Autodesk Inventor part; units mm, degrees
ref_plane "YZ Plane" through (0, 0, 0) normal (1, 0, 0) x (0, 1, 0)
ref_plane "XZ Plane" through (0, 0, 0) normal (0, 1, 0) x (-1, 0, 0)
ref_plane "XY Plane" through (0, 0, 0) normal (0, 0, 1) x (1, 0, 0)
sketch "Sketch1" plane through (0, 0, 0) normal (0, 0, 1) x (1, 0, 0)
  line L0 (0, 40) -> (34.641, -20)
  line L1 (34.641, -20) -> (-34.641, -20)
  line L2 (-34.641, -20) -> (0, 40)
  circle A0 centre (0, 0) radius 1
  dimension "d0" = 2
  dimension "d1" = 20
extrude "Extrusion1" add sketch "Sketch1" along normal blind 5.66
sketch "Sketch2" plane through (0, 0, 5.66) normal (0, 0, 1) x (1, 0, 0)
  circle A0 centre (0, 0) radius 1
  line L0 (-34.641, -20) -> (34.641, -20)
  line L1 (0, -1) -> (0, 0)
  line L2 (-2.83, -11.66) -> (-2.83, -20)
  line L3 (2.83, -11.66) -> (2.83, -20)
  line L4 (2.83, -11.66) -> (-2.83, -11.66)
  point P0 (0, -20)
  dimension "d15" = 8.34
  dimension "d16" = 2.83
  dimension "d17" = 2.83
extrude "Extrusion2" cut sketch "Sketch2" against normal blind 8.625
pattern_circular "Circular Pattern1" count 3 over 360 about axis through (0, 0, 0) along (0, 0, 1) of "Extrusion2"
chamfer "Chamfer1" distance 10 angle 45 3 edges at (34.641, -20, 2.83) (-34.641, -20, 2.83) (0, 40, 2.83)
fillet "Fillet1" radius 2 6 edges at (-29.641, -11.3397, 2.83) (-24.641, -20, 2.83) (-5, 31.3397, 2.83) (5, 31.3397, 2.83) (29.641, -11.3397, 2.83) (24.641, -20, 2.83)
properties part number "Lower Platform"
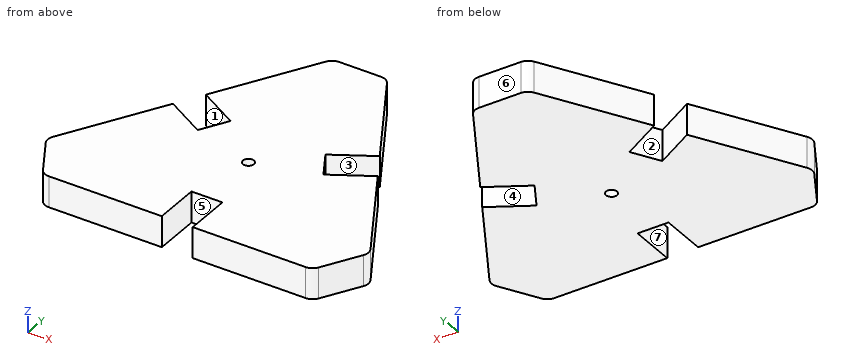
Design review of the part built by this model. Coordinates are the model's own, in mm. Face numbers are marked on the shaded views. A direction names the side the tool comes from. Give positions to 0.01 mm unless a question says otherwise; leave off trailing zeros. Loops run counter-clockwise (first coordinate to the right, second up) from the corner with the lowest first, then second, coordinate; pieces in that order, holes last. Notation, with made-up numbers: (29.5, -34) - (58.5, -34) arc R25 ccw to (58.5, -21) - close; hole circle Ø8 at (-25, -36.75). An arc over 180 degrees is marked (long way). Write item = value, one per line.
1) To check wall thickness, follow line 1 (Y direction, x = 0, z = 1.95); line 2 (X direction, y = -12.5, z = 1.4); line 3 (X direction, y = 0, z = 3.85). State the ranges of each line that lie inside material, in increasing order.
Result sheet:
line_1 = -11.66 to -1, 1 to 31.34
line_2 = -28.97 to -2.83, 2.83 to 28.97
line_3 = -23.09 to -1, 1 to 23.09
2) Take a section at A-A on x = 0. State the section outline as (y, z) points, and give its area (3 significant figures).
Result sheet:
outline = (-11.66, 0) - (-1, 0) - (-1, 5.66) - (-11.66, 5.66) - close; (1, 0) - (31.34, 0) - (31.34, 5.66) - (1, 5.66) - close
area = 232 mm2
3) Draft analysis for pull direction Y (two halves, no side actions). For the marked faces 4, 5, 6 and 7, state which applies: +Y half, -Y half, draft (parallel to the pull), parting line (faces both ways), or undercut.
Result sheet:
face_4 = undercut
face_5 = -Y half
face_6 = +Y half
face_7 = draft
4) Take a section at D-D on y = 27. State the section outline as (x, z) points, and give its area (3 significant figures).
Result sheet:
outline = (-7.51, 0) - (7.51, 0) - (7.51, 5.66) - (-7.51, 5.66) - close
area = 85.0 mm2
5) Take a section at B-B on y = 0. State the section outline as (x, z) points, and give its area (3 significant figures).
Result sheet:
outline = (-23.09, 0) - (-1, 0) - (-1, 5.66) - (-23.09, 5.66) - close; (1, 0) - (23.09, 0) - (23.09, 5.66) - (1, 5.66) - close
area = 250 mm2
6) Tool access review of the marked faces 1, 2 and 3: name each direction out of +Z, -Z, +X, -X, +Y, -Y from which nothing blocks a thin tool from reaching the whole face with its end or side.
Result sheet:
face_1 = +Z, -Z, -X
face_2 = +Z, -Z
face_3 = +Z, -Z, +X
7) Take a section at C-C on z = 1.7. State the section outline as (x, y) points.
Result sheet:
outline = (-29.06, -12.34) - (-25.22, -19) arc R2 ccw to (-23.49, -20) - (-2.83, -20) - (-2.83, -11.66) - (2.83, -11.66) - (2.83, -20) - (23.49, -20) arc R2 ccw to (25.22, -19) - (29.06, -12.34) arc R2 ccw to (29.06, -10.34) - (18.74, 7.55) - (11.51, 3.38) - (8.68, 8.28) - (15.91, 12.45) - (5.58, 30.34) arc R2 ccw to (3.85, 31.34) - (-3.85, 31.34) arc R2 ccw to (-5.58, 30.34) - (-15.91, 12.45) - (-8.68, 8.28) - (-11.51, 3.38) - (-18.74, 7.55) - (-29.06, -10.34) arc R2 ccw to start; hole circle Ø2 at (0, 0)
8) Clearance check with flat-ended pins moving along their axes: pin 1 Ø1.7 at (y, z) = (-14.5, 3.5) entering from -X; pin 2 Ø1.7 at (x, z) = (-0.5, 2) entering from -Y; pin 3 Ø1.5 at (x, z) = (20.5, 4.5) entering from +Y; pin 4 Ø1.8 at (x, y) = (0, 0) entering from +Z. State where each tip first meets the part, or that it passes through.
Result sheet:
pin_1 = -28.31
pin_2 = -11.66
pin_3 = 5.79
pin_4 = through
